```python
from build123d import *

# Parameters (mm, degrees)
F0_W     = 57.4
F0_H     = 57.4
F0_W_2   = 55
F0_H_2   = 55
F1_DEPTH = 20
F2_W     = 65
F2_H     = 65
F2_W_2   = 57.4
F2_H_2   = 57.4
F3_DEPTH = 5


with BuildPart() as f1:
    # F0 (on Top) → F1 (new body)
    with BuildSketch(Plane.XY):
        with Locations((28.7, 28.7)):
            Rectangle(F0_W, F0_H)
        with Locations((28.7, 28.7)):
            Rectangle(F0_W_2, F0_H_2, mode=Mode.SUBTRACT)
    extrude(amount=F1_DEPTH)

    # F2 (on face) → F3 (join)
    with BuildSketch(Plane.XY.offset(20)):
        with Locations((28.7, 28.7)):
            Rectangle(F2_W, F2_H)
        with Locations((28.7, 28.7)):
            Rectangle(F2_W_2, F2_H_2, mode=Mode.SUBTRACT)
    extrude(amount=-F3_DEPTH)


solid = f1.part
```
Read the model definition and answer for the solid it produces. Units are mm, in the model's axes. A direction names the side the tool comes from. Give positions to 0.01 mm unless a question says otherwise; leave off trailing zeros. Loops run counter-clockwise (first coordinate to the right, second up) from the corner with the lowest first, then second, coordinate; pieces in that order, holes last.
Item 1: For faces 1 (the flat face through (57.4, 28, 7)), 2 (the flat face through (28, 0, 7)), 3 (the flat face through (0, 28, 7)), 4 (the flat face through (28, 57.4, 7)), 5 (the flat face through (1.2, 28, 10)), determine the directions among +Z, -Z, +X, -X, +Y, -Y from which every point of the face is accessible in a straight line to the end or side of a thin tool.
Item 2: The part is cut by section B-B (z = 12). Write down the section's boundary in (x, y).
Item 3: The part is cut by section A-A (x = 22). Write down the section's boundary in (y, z), and give its area (3 significant figures).
Item 4: The part is cut by section D-D (z = 17.5). Write down the section's boundary in (x, y).
Item 5: The mould has two halves that part along Y. Classify faces 6 (the flat face through (28, 61.2, 18)), 7 (the flat face through (56.2, 28, 10)), 8 (the flat face through (28, 0, 20)), 9 (the flat face through (28, -3.8, 18)): released by +Y, released by -Y, zero draft, split by the parting line, or undercut.
Item 6: Each of these flat-tipped pins is pushed along its axis until it touches: pin 1 Ø3 at (x, z) = (54, 4) entering from -Y; pin 2 Ø6 at (x, z) = (8, 13) entering from -Y; pin 3 Ø8 at (y, z) = (35.5, 6.5) entering from +X; pin 4 Ø7.5 at (x, z) = (39.5, 6.5) entering from +Y. Where does it stop, or does it pass through?
Item 7: Find the intervals of material crossed by line 1 along Y through (x, z) = (35, 19); line 2 along Y through (x, z) = (30, 9.75), in increasing order.
Taken from the geometry:
1. face 1: -Z, +X, +Y, -Y
1. face 2: -Z, +X, -X, -Y
1. face 3: -Z, -X, +Y, -Y
1. face 4: -Z, +X, -X, +Y
1. face 5: +Z, -Z
2. outline: (0, 0) - (57.4, 0) - (57.4, 57.4) - (0, 57.4) - close; hole (1.2, 1.2) - (56.2, 1.2) - (56.2, 56.2) - (1.2, 56.2) - close
3. outline: (-3.8, 15) - (0, 15) - (0, 0) - (1.2, 0) - (1.2, 20) - (-3.8, 20) - close; (56.2, 0) - (57.4, 0) - (57.4, 15) - (61.2, 15) - (61.2, 20) - (56.2, 20) - close
3. area: 86.0 mm2
4. outline: (-3.8, -3.8) - (61.2, -3.8) - (61.2, 61.2) - (-3.8, 61.2) - close; hole (1.2, 1.2) - (56.2, 1.2) - (56.2, 56.2) - (1.2, 56.2) - close
5. face 6: released by +Y
5. face 7: undercut
5. face 8: zero draft
5. face 9: released by -Y
6. pin 1: stops at y = 0
6. pin 2: stops at y = -3.8
6. pin 3: stops at x = 57.4
6. pin 4: stops at y = 57.4
7. line 1: y = -3.8 to 1.2, 56.2 to 61.2
7. line 2: y = 0 to 1.2, 56.2 to 57.4
